Solid Edge part; units mm, degrees
sketch "Sketch1" plane through (0, 0, 0) normal (0, -1, 0) x (1, 0, 0)
  line L0 (0, 23) -> (25, 23)
  line L1 (25, 23) -> (25, 0)
  line L2 (25, 0) -> (0, 0)
  line L3 (0, 0) -> (0, 23)
extrude "Protrusion1" add sketch "Sketch1" against normal blind 30
sketch "Sketch2" plane through (0, 15, 11.5) normal (-1, 0, 0) x (0, -1, 0)
  line L0 (13, 5.7235) -> (-13, 5.7235)
  line L1 (-13, 5.7235) -> (-13, 7.7235)
  line L2 (-13, 7.7235) -> (13, 7.7235)
  line L3 (13, 7.7235) -> (13, 5.7235)
extrude "ExtrudedCutout_2" cut sketch "Sketch2" against normal blind 20
sketch "Sketch3" plane through (12.5, 15, 23) normal (0, 0, 1) x (0, -1, 0)
  circle A0 centre (0, 2.5) radius 1.5
extrude "ExtrudedCutout_3" cut sketch "Sketch3" against normal blind 10
sketch "Sketch4" plane through (0, 15, 11.5) normal (-1, 0, 0) x (0, -1, 0)
  line L0 (9, 0.7235) -> (-9, 0.7235)
  line L1 (-9, 0.7235) -> (-9, -14.6264)
  line L2 (-9, -14.6264) -> (9, -14.6264)
  line L3 (9, -14.6264) -> (9, 0.7235)
extrude "ExtrudedCutout_4" cut sketch "Sketch4" against normal blind 84.6021
fillet "Round_2" radius 1 4 edges at (12.5, 0, 23) (12.5, 0, 0) (12.5, 30, 23) (12.5, 30, 0)
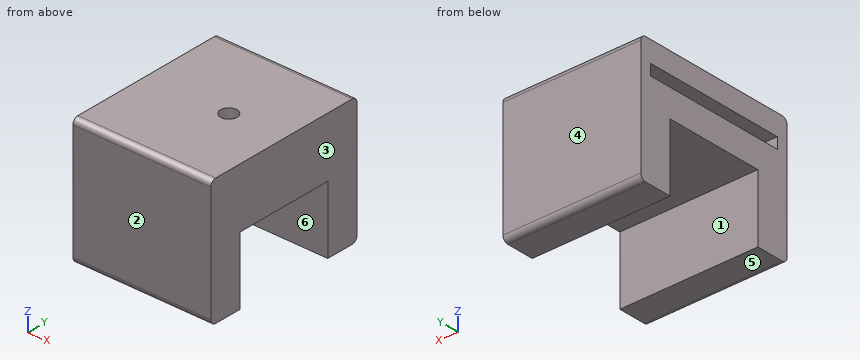
Here's how the part is built. I have some questions about the finished solid (model axes, mm). Face numbers are marked on the shaded views. A direction names the side the tool comes from. Round coordinates to 2 decimals unless told otherwise and drop trailing zeros. Loops run counter-clockwise (first coordinate to the right, second up) from the corner with the lowest first, then second, coordinate; pieces in that order, holes last. Notation, with made-up numbers: (13, -27.75) -> (27, -27.75) arc R9 cw to (27, -16.75) -> close; hole circle Ø2 at (-18, -3.5). An arc over 180 degrees is marked (long way). Answer as CSV lines item,"result". Start each with the question number.
1. Imagine slicing it at C-C on x = 5. Write out the boundary of the cut face in (y, z), plus the area to 3 significant figures.
2. Imagine slicing it at D-D on y = 11.75. Write out the boundary of the cut face in (x, z), plus the area to 3 significant figures.
3. I need wall thicknesses on probe 1 along Z at (x, y) = (5.75, 12.5); probe 2 along X at (y, z) = (15, 22.2); probe 3 along Y at (x, z) = (4, 17.75). Which ranges of each line are inside material? Lowest first, please. Write a range as from..to.
4. I'm going to push flat-ended pins straight in: P1, Ø1.8, axis at x = 15, y = 15, coming from the +Z side; P2, Ø12, axis at x = 15, y = 14, coming from the -Z side; P3, Ø0.6, axis at y = 15, z = 18.5, coming from the -X side. Where does each tip first touch, or does it pass through?
5. Imagine slicing it at B-B on z = 3.5. Write out the boundary of the cut face in (x, y), plus the area to 3 significant figures.
6. If we mould it in two halves opening along Y, with no side actions, what happens to the marked faces 1, 2, 3 and 4? For each: pulls with the +Y half, pulls with the -Y half, needs draft (parallel to the pull), parting line crosses it, or undercut.
7. For the marked faces 5 and 6, which set-ups out of +Z, -Z, +X, -X, +Y, -Y let a thin tool reach every point of the face, with its end or its side?
8. Imagine slicing it at A-A on y = 15. Write out the boundary of the cut face in (x, z), plus the area to 3 significant figures.
Solution:
1,outline,"(0, 1) arc R1 ccw to (1, 0) -> (6, 0) -> (6, 12.22) -> (24, 12.22) -> (24, 0) -> (29, 0) arc R1 ccw to (30, 1) -> (30, 22) arc R1 ccw to (29, 23) -> (1, 23) arc R1 ccw to (0, 22) -> close; hole (2, 17.22) -> (28, 17.22) -> (28, 19.22) -> (2, 19.22) -> close"
1,area,"417 mm²"
2,outline,"(0, 12.22) -> (25, 12.22) -> (25, 23) -> (0, 23) -> (0, 19.22) -> (20, 19.22) -> (20, 17.22) -> (0, 17.22) -> close"
2,area,"229 mm²"
3,probe 1,"12.22..17.22, 19.22..23"
3,probe 2,"0..13.5, 16.5..25"
3,probe 3,"0..2, 28..30"
4,P1,"z = 13"
4,P2,"z = 12.22"
4,P3,"x = 20"
5,outline,"(0, 0) -> (25, 0) -> (25, 6) -> (0, 6) -> close; (0, 24) -> (25, 24) -> (25, 30) -> (0, 30) -> close"
5,area,"300 mm²"
6,face 1,"undercut"
6,face 2,"pulls with the -Y half"
6,face 3,"needs draft"
6,face 4,"pulls with the +Y half"
7,face 5,"-Z, +X, -X, +Y, -Y"
7,face 6,"-Z, +X, -X"
8,outline,"(0, 12.22) -> (25, 12.22) -> (25, 23) -> (16.5, 23) -> (16.5, 19.22) -> (20, 19.22) -> (20, 17.22) -> (16.5, 17.22) -> (16.5, 13) -> (13.5, 13) -> (13.5, 17.22) -> (0, 17.22) -> close; (0, 19.22) -> (13.5, 19.22) -> (13.5, 23) -> (0, 23) -> close"
8,area,"205 mm²"
